Check sheet for the modelled part. Datum: model origin and axes. Units: mm. Coordinates: 2 decimals unless noted, no trailing zeros. Loops run counter-clockwise (first coordinate to the right, second up) from the corner with the lowest first, then second, coordinate; pieces in that order, holes last. Notation, with made-up numbers: (86, 28) - (118, 28) arc R19 ccw to (118, 47) - close; hole circle Ø2 at (-11.75, 17.25). An arc over 180 degrees is marked (long way). Answer as a JSON object with one key per item and string values. Group by question number.
from build123d import *

# Parameters (mm, degrees)
SKETCH2_R           = 4.85
BOSS_EXTRUDE1_DEPTH = 4.5
SKETCH3_W           = 0.45
SKETCH3_H           = 0.35
BOSS_EXTRUDE2_DEPTH = 4.5


with BuildPart() as part:
    # Sketch2 → Boss-Extrude1 (new body)
    with BuildSketch(Plane.XY):
        Circle(SKETCH2_R)
    extrude(amount=BOSS_EXTRUDE1_DEPTH)

    # Sketch3 → Boss-Extrude2 (add)
    with BuildSketch(Plane.XY.offset(4.5)):
        with Locations((-1.25, 0)):
            Rectangle(SKETCH3_W, SKETCH3_H)
        with Locations((1.25, 0)):
            Rectangle(SKETCH3_W, SKETCH3_H)
    extrude(amount=BOSS_EXTRUDE2_DEPTH)


solid = part.part
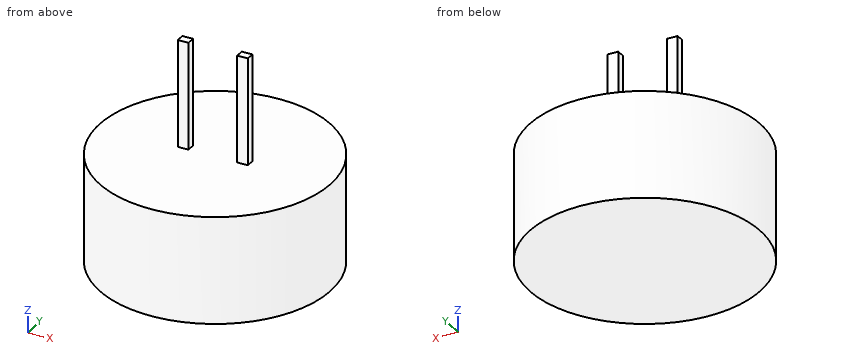
1. Material ranges on line 1 (Z direction, x = -3.25, y = 2.5); line 2 (Y direction, x = 1.25, z = 5) (3 decimals); line 3 (Y direction, x = 2.25, z = 3), recorded low to high.
2. Gauge pin test, flat ends, axial feed: pin 1 (1 mm diameter, centred on y = -1, z = 1, fed in from -X); pin 2 (0.5 mm diameter, centred on x = 1, z = 5.5, fed in from -Y) (3 decimals); pin 3 (4 mm diameter, centred on x = -2.5, z = 3, fed in from +Y). Record the tip position at first contact, or that the pin passes through.
3. Sectioned sample at D-D on z = 2.5. Record the cut outline in (x, y), plus the area to 3 significant figures.
4. Sectioned sample at C-C on x = 1.25. Record the cut outline in (y, z) (3 decimals), plus the area to 3 significant figures.
5. Sectioned sample at B-B on y = 0. Record the cut outline in (x, z) (3 decimals).
6. Sectioned sample at A-A on z = 7. Record the cut outline in (x, y) (3 decimals), plus the area to 3 significant figures.
Answers follow:
{
 "1": {"line 1": "z = 0 to 4.5", "line 2": "y = -0.175 to 0.175", "line 3": "y = -4.3 to 4.3"},
 "2": {"pin 1": "stops at x = -4.82", "pin 2": "stops at y = -0.175", "pin 3": "stops at y = 4.82"},
 "3": {"outline": "circle Ø9.7 at (0, 0)", "area": "73.9 mm^2"},
 "4": {"outline": "(-4.686, 0) - (4.686, 0) - (4.686, 4.5) - (0.175, 4.5) - (0.175, 9) - (-0.175, 9) - (-0.175, 4.5) - (-4.686, 4.5) - close", "area": "43.8 mm^2"},
 "5": {"outline": "(-4.85, 0) - (4.85, 0) - (4.85, 4.5) - (1.475, 4.5) - (1.475, 9) - (1.025, 9) - (1.025, 4.5) - (-1.025, 4.5) - (-1.025, 9) - (-1.475, 9) - (-1.475, 4.5) - (-4.85, 4.5) - close"},
 "6": {"outline": "(-1.475, -0.175) - (-1.025, -0.175) - (-1.025, 0.175) - (-1.475, 0.175) - close; (1.025, -0.175) - (1.475, -0.175) - (1.475, 0.175) - (1.025, 0.175) - close", "area": "0.315 mm^2"}
}
